Geometry check sheet. Reference: the model listing, model coordinates, mm. A direction names the side the tool comes from. Round coordinates to 2 decimals unless told otherwise and drop trailing zeros. Order: outer loops, then holes, each group sorted by start corner. A loop starts at its lowest first (then second) coordinate and runs counter-clockwise, first axis right, second up. Notation, with made-up numbers: (-38.5, 26.25) - (-22.5, 26.25) arc R21 ccw to (-22.5, 31.25) - close; hole circle Ø1 at (-29, 55.25). An arc over 180 degrees is marked (long way). Return JSON: item names as keys, results as strings. Group by question number.
Q1. Tool access check on faces 1 (the flat face through (11, -15, 18.3)), 2 (the flat face through (13, -4, 12)), 3 (the flat face through (15, -28, 12)), 4 (the flat face through (6, -15, 24)), 5 (the flat face through (14, -4.5, 12)). Record the directions out of +Z, -Z, +X, -X, +Y, -Y that give a thin tool (end or side, any length) a straight path to the whole face; none if there is none.
Q2. Sectioned sample at C-C, the plane z = 16.25. Record the cut outline in (x, y), then the cut area to 3 significant figures.
Q3. Sectioned sample at A-A, the plane y = -26.5. Record the cut outline in (x, z), then the cut area to 3 significant figures.
Q4. Material ranges on line 1 along X through (y, z) = (-26.5, 2.5); line 2 along Y through (x, z) = (12.25, 16); line 3 along Y through (x, z) = (13.5, 1.25), recorded low to high.
Q5. Sectioned sample at D-D, the plane x = 9.75. Record the cut outline in (y, z), then the cut area to 4 significant figures.
Q6. Draft check along X on faces 6 (the flat face through (12, -27.5, 15)), 7 (the flat face through (14, -25.5, 12)), 8 (the flat face through (15, -2, 12)). Enter one of: pulls with the +X half, pulls with the -X half, needs draft (parallel to the pull), parting line crosses it, or undercut.
Q7. Sectioned sample at B-B, the plane x = 13.75. Record the cut outline in (y, z), then the cut area to 3 significant figures.
Q8. Gauge pin test, flat ends, axial feed: pin 1 Ø5.5 at (y, z) = (-18, 10.5) entering from +X; pin 2 Ø1.6 at (y, z) = (-3.5, 14) entering from -X; pin 3 Ø3 at (x, y) = (11, -14.5) entering from +Z. Record the tip position at first contact, or that the pin passes through.
```python
from build123d import *

# Parameters (mm, degrees)
F0_W     = 15
F0_H     = 24
F1_DEPTH = 30
F2_W     = 1.2
F2_H     = 25
F3_DEPTH = 24.001
F4_W     = 2
F4_H     = 21
F5_DEPTH = 24.001
F6_W     = 2.5
F6_H     = 25
F7_DEPTH = 5.7


with BuildPart() as f1:
    # F0 (on Front) → F1 (new body)
    with BuildSketch(Plane.XZ):
        with Locations((7.5, 12)):
            Rectangle(F0_W, F0_H)
    extrude(amount=F1_DEPTH)

    # F2 (on face) → F3 (cut, through all)
    with BuildSketch(Plane.XY.offset(24)):
        with Locations((12.4, -15)):
            Rectangle(F2_W, F2_H)
    extrude(amount=-F3_DEPTH, mode=Mode.SUBTRACT)

    # F4 (on face) → F5 (cut, through all)
    with BuildSketch(Plane.XY.offset(24)):
        with Locations((14, -15)):
            Rectangle(F4_W, F4_H)
    extrude(amount=-F5_DEPTH, mode=Mode.SUBTRACT)

    # F6 (on face) → F7 (cut)
    with BuildSketch(Plane.XY.offset(24)):
        with Locations((10.55, -15)):
            Rectangle(F6_W, F6_H)
    extrude(amount=-F7_DEPTH, mode=Mode.SUBTRACT)


solid = f1.part
```
Reply:
{
 "1": {"face 1": "+Z", "face 2": "+Z, -Z", "face 3": "+Z, -Z, +X, +Y, -Y", "face 4": "+Z, +X, -X, +Y, -Y", "face 5": "+Z, -Z, +X"},
 "2": {"outline": "(0, -30) - (15, -30) - (15, -25.5) - (13, -25.5) - (13, -27.5) - (11.8, -27.5) - (11.8, -2.5) - (13, -2.5) - (13, -4.5) - (15, -4.5) - (15, 0) - (0, 0) - close", "area": "378 mm^2"},
 "3": {"outline": "(0, 0) - (11.8, 0) - (11.8, 18.3) - (9.3, 18.3) - (9.3, 24) - (0, 24) - close; (13, 0) - (15, 0) - (15, 24) - (13, 24) - close", "area": "317 mm^2"},
 "4": {"line 1": "0 to 11.8, 13 to 15", "line 2": "-30 to -27.5, -2.5 to 0", "line 3": "-30 to -25.5, -4.5 to 0"},
 "5": {"outline": "(-30, 0) - (0, 0) - (0, 24) - (-2.5, 24) - (-2.5, 18.3) - (-27.5, 18.3) - (-27.5, 24) - (-30, 24) - close", "area": "577.5 mm^2"},
 "6": {"face 6": "undercut", "face 7": "needs draft", "face 8": "pulls with the +X half"},
 "7": {"outline": "(-30, 0) - (-25.5, 0) - (-25.5, 24) - (-30, 24) - close; (-4.5, 0) - (0, 0) - (0, 24) - (-4.5, 24) - close", "area": "216 mm^2"},
 "8": {"pin 1": "x = 11.8", "pin 2": "x = 0", "pin 3": "z = 18.3"}
}
